Check sheet for the modelled part. Datum: model origin and axes. Units: mm. A direction names the side the tool comes from. Coordinates: 2 decimals unless noted, no trailing zeros. Order: outer loops, then holes, each group sorted by start corner. A loop starts at its lowest first (then second) coordinate and runs counter-clockwise, first axis right, second up.
1. Gauge pin test, flat ends, axial feed: pin 1 Ø12 at (y, z) = (-24, 272) entering from +X; pin 2 Ø2 at (x, z) = (-313.5, 39) entering from -Y; pin 3 Ø5 at (x, y) = (-316, -41.5) entering from -Z. Record the tip position at first contact, or that the pin passes through.
2. Draft check along X on faces 1 (the cylindrical face through (-263.54, 17.12, 46.76)), 2 (the flat face through (-320, 17, 160)), 3 (the flat face through (-233, -35.27, 196)). Enter one of: released by +X, released by -X, zero draft, split by the parting line, or undercut.
3. Cross-section at B-B (z = 89.5). Enter the section's corners in (x, y), then the cut area to 3 significant figures.
4. Cross-section at A-A (x = -285). Enter the section's corners in (y, z), then the cut area to 3 significant figures.
5. Cross-section at D-D (x = -35). Enter the section's corners in (y, z), then the cut area to 3 significant figures.
6. Cross-section at C-C (z = 40). Enter the section's corners in (x, y).
7. Set-up check for faces 4 (the flat face through (-281, 17, 0)), 5 (the flat face through (-229, -20.27, 196)), 6 (the flat face through (0, -28, 284)): record each of +Z, -Z, +X, -X, +Y, -Y from which the full face is reachable in a straight line by a thin tool's end or side.
8. Thickness scan on line 1 (Y direction, x = -285.5, z = 293); line 2 (Z direction, x = -285, y = 13); line 3 (Z direction, x = -70.5, y = -7.5). Record the ranges inside material, lowest first.
```python
from build123d import *

# Parameters (mm, degrees)
F0_W     = 320
F0_H     = 60
F1_DEPTH = 360
F2_R     = 22.5
F3_DEPTH = 60
F5_DEPTH = 60
F6_W     = 403.911207
F6_H     = 133.211269
F6_W_2   = 320
F6_H_2   = 60
F7_DEPTH = 35
F8_W     = 30
F8_H     = 325
F9_DEPTH = 320


with BuildPart() as f1:
    # F0 (on Top) → F1 (new body)
    with BuildSketch(Plane.XY):
        with Locations((-160, -5.27027)):
            Rectangle(F0_W, F0_H)
    extrude(amount=F1_DEPTH)

    # F2 (on face) → F3 (cut, through all)
    with BuildSketch(Plane.XZ.offset(35.27027)):
        with Locations((-285, 40)):
            Circle(F2_R)
        with Locations((-35, 290)):
            Circle(F2_R)
        with Locations((-205, 245)):
            Circle(F2_R)
    extrude(amount=-F3_DEPTH, mode=Mode.SUBTRACT)

    # F4 (on face) → F5 (cut, through all)
    with BuildSketch(Plane.XZ.offset(35.27027)):
        Polygon((0, 243.859082), (-27.186546, 30.584865), (-240, 0), (0, 0), align=None)
        with BuildLine():
            Line((-240, 0), (-27.186546, 30.584865))
            Line((-27.186546, 30.584865), (0, 243.859082))
            ThreePointArc((0, 243.859082), (-180.42215, 181.395507), (-240, 0))
        make_face()
    extrude(amount=-F5_DEPTH, mode=Mode.SUBTRACT)

    # F6 (on face) → F7 (join)
    with BuildSketch(Plane.XY.offset(360)):
        with Locations((-158.057762, -2.021872)):
            Rectangle(F6_W, F6_H)
        with Locations((-160, -5.27027)):
            Rectangle(F6_W_2, F6_H_2, mode=Mode.SUBTRACT)
    extrude(amount=-F7_DEPTH)

    # F8 (on face) → F9 (cut, through all)
    with BuildSketch(Plane.YZ):
        with Locations((-5.27027, 162.5)):
            Rectangle(F8_W, F8_H)
    extrude(amount=-F9_DEPTH, mode=Mode.SUBTRACT)


solid = f1.part
```
Data:
1. pin 1: stops at x = 0
1. pin 2: stops at y = -35.27
1. pin 3: stops at z = 325
2. face 1: undercut
2. face 2: released by -X
2. face 3: zero draft
3. outline: (-320, -35.27) - (-233.96, -35.27) - (-233.96, -20.27) - (-320, -20.27) - close; (-320, 9.73) - (-233.96, 9.73) - (-233.96, 24.73) - (-320, 24.73) - close
3. area: 2,580 mm2
4. outline: (-68.63, 325) - (-35.27, 325) - (-35.27, 62.5) - (-20.27, 62.5) - (-20.27, 325) - (9.73, 325) - (9.73, 62.5) - (24.73, 62.5) - (24.73, 325) - (64.58, 325) - (64.58, 360) - (-68.63, 360) - close; (-35.27, 0) - (-20.27, 0) - (-20.27, 17.5) - (-35.27, 17.5) - close; (9.73, 0) - (24.73, 0) - (24.73, 17.5) - (9.73, 17.5) - close
4. area: 13,100 mm2
5. outline: (-68.63, 325) - (-35.27, 325) - (-35.27, 312.5) - (-20.27, 312.5) - (-20.27, 325) - (9.73, 325) - (9.73, 312.5) - (24.73, 312.5) - (24.73, 325) - (64.58, 325) - (64.58, 360) - (-68.63, 360) - close; (-35.27, 245.44) - (-20.27, 245.44) - (-20.27, 267.5) - (-35.27, 267.5) - close; (9.73, 245.44) - (24.73, 245.44) - (24.73, 267.5) - (9.73, 267.5) - close
5. area: 5,700 mm2
6. outline: (-320, -35.27) - (-307.5, -35.27) - (-307.5, -20.27) - (-320, -20.27) - close; (-320, 9.73) - (-307.5, 9.73) - (-307.5, 24.73) - (-320, 24.73) - close; (-262.5, -35.27) - (-241.98, -35.27) - (-241.98, -20.27) - (-262.5, -20.27) - close; (-262.5, 9.73) - (-241.98, 9.73) - (-241.98, 24.73) - (-262.5, 24.73) - close
7. face 4: -Z, +X, -X, +Y, -Y
7. face 5: -Z, +X, -X
7. face 6: -Z, +X, +Y, -Y
8. line 1: y = -35.27 to -20.27, 9.73 to 24.73
8. line 2: z = 0 to 17.5, 62.5 to 360
8. line 3: z = 325 to 360
